from build123d import *

# Parameters (mm, degrees)
F0_W     = 38.296241
F0_H     = 31.86328
F1_DEPTH = 25.4
F2_W     = 25.530826
F2_H     = 31.86328
F3_DEPTH = 6.35
F4_W     = 25.530827
F4_H     = 31.86328
F5_DEPTH = 6.35


with BuildPart() as f1:
    # F0 (on Front) → F1 (new body)
    with BuildSketch(Plane.XZ):
        with Locations((19.14812, 15.93164)):
            Rectangle(F0_W, F0_H)
    extrude(amount=F1_DEPTH)

    # F2 (on face) → F3 (cut)
    with BuildSketch(Plane.XZ.offset(25.4)):
        with Locations((25.530828, 15.93164)):
            Rectangle(F2_W, F2_H)
    extrude(amount=-F3_DEPTH, mode=Mode.SUBTRACT)

    # F4 (on face) → F5 (cut)
    with BuildSketch(Plane(origin=(0, 0, 0), x_dir=(-1, 0, 0), z_dir=(0, 1, 0))):
        with Locations((-25.530827, 15.93164)):
            Rectangle(F4_W, F4_H)
    extrude(amount=-F5_DEPTH, mode=Mode.SUBTRACT)


solid = f1.part
Build history of the part. All positions in model axes, mm. A direction names the side the tool comes from. Round coordinates to 2 decimals unless told otherwise and drop trailing zeros. Loops run counter-clockwise (first coordinate to the right, second up) from the corner with the lowest first, then second, coordinate; pieces in that order, holes last. Notation, with made-up numbers: (49.25, 30.5) -> (66.25, 30.5) arc R19 ccw to (66.25, 54.5) -> close; hole circle Ø8 at (26.5, -7.5). An arc over 180 degrees is marked (long way). Answer in a Markdown table with one row per item.
Item 1: Saw through at C-C (y = -1.75). Write the cut outline in (x, z), and give its area (3 significant figures).
Answers below:
| item | result |
|---|---|
| outline | (0, 0) -> (12.77, 0) -> (12.77, 31.86) -> (0, 31.86) -> close |
| area | 407 mm² |
Item 2: Which spindle directions (+Z, -Z, +X, -X, +Y, -Y) get a long thin tool onto all of the face, cutting with end or side? Do faces 1 (the flat face through (12.765, -22, 16)), 2 (the flat face through (12.765, -3, 16)), 3 (the flat face through (15, -13, 0)). Say none if no direction does.
Answers below:
| item | result |
|---|---|
| face 1 | +Z, -Z, +X, -Y |
| face 2 | +Z, -Z, +X, +Y |
| face 3 | -Z, +X, -X, +Y, -Y |
Item 3: Saw through at B-B (x = 17). Write the cut outline in (y, z), and give its area (3 significant figures).
Answers below:
| item | result |
|---|---|
| outline | (-19.05, 0) -> (-6.35, 0) -> (-6.35, 31.86) -> (-19.05, 31.86) -> close |
| area | 405 mm² |
Item 4: Saw through at A-A (z = 12). Write the cut outline in (x, y).
Answers below:
| item | result |
|---|---|
| outline | (0, -25.4) -> (12.77, -25.4) -> (12.77, -19.05) -> (38.3, -19.05) -> (38.3, -6.35) -> (12.77, -6.35) -> (12.77, 0) -> (0, 0) -> close |
Item 5: Pin check, flat tips, straight feed: pin 1 (5 mm diameter, centred on y = -2, z = 17.5, fed in from +X); pin 2 (12 mm diameter, centred on x = 10, z = 8, fed in from +Y); pin 3 (1 mm diameter, centred on x = 23.5, z = 4.5, fed in from -Y). Stop position of each tip, or through.
Answers below:
| item | result |
|---|---|
| pin 1 | stops at x = 12.77 |
| pin 2 | stops at y = 0 |
| pin 3 | stops at y = -19.05 |
Item 6: Drill centre lines: L1, parallel to Y at x = 17.5, z = 26; L2, parallel to X at y = -1.25, z = 22. Where is each one in solid material? Low to high. Write a range as [from, to].
Answers below:
| item | result |
|---|---|
| L1 | y = [-19.05, -6.35] |
| L2 | x = [0, 12.77] |
